```python
from build123d import *

# Parameters (mm, degrees)
SKETCH1_R           = 2.1
BOSS_EXTRUDE1_DEPTH = 5
SKETCH3_W           = 30
SKETCH3_H           = 5
BOSS_EXTRUDE2_DEPTH = 15
FILLET1_R           = 5
SKETCH4_R           = 2.6
CUT_EXTRUDE2_DEPTH  = 108.425323176
FILLET2_R           = 10
SKETCH5_R           = 4.4
CUT_EXTRUDE3_DEPTH  = 108.425323272
SKETCH2_R           = 3.6
CUT_EXTRUDE4_DEPTH  = 114.974558916


with BuildPart() as part:
    # Sketch1 → Boss-Extrude1 (new body)
    with BuildSketch(Plane.XY):
        Polygon((73.634936481, -21), (73.634936481, -20), (103.634936481, -20), (103.634936481, -21), (103.634936481, -45), (73.634936481, -45), align=None)
        with Locations((98.634936481, -35.1)):
            Circle(SKETCH1_R, mode=Mode.SUBTRACT)
        with Locations((78.634936481, -35.1)):
            Circle(SKETCH1_R, mode=Mode.SUBTRACT)
        with Locations((98.634936481, -25.1)):
            Circle(SKETCH1_R, mode=Mode.SUBTRACT)
        with Locations((78.634936481, -25.1)):
            Circle(SKETCH1_R, mode=Mode.SUBTRACT)
    extrude(amount=BOSS_EXTRUDE1_DEPTH)

    # Sketch3 → Boss-Extrude2 (add)
    with BuildSketch(Plane.XY.offset(5)):
        with Locations((88.634936481, -42.5)):
            Rectangle(SKETCH3_W, SKETCH3_H)
    extrude(amount=BOSS_EXTRUDE2_DEPTH)

    # Fillet1
    fillet1_edges = [part.edges().sort_by_distance(p)[0] for p in [
        (103.634936481, -20, 2.5),
        (73.634936481, -20, 2.5),
    ]]
    fillet(fillet1_edges, radius=FILLET1_R)

    # Sketch4 → Cut-Extrude2 (cut, through all)
    with BuildSketch(Plane(origin=(0, -40, 0), x_dir=(1, 0, 0), z_dir=(0, 1, 0))):
        with Locations(Location((88.634936481, -12.5, 0), (0, 0, 180))):
            Circle(SKETCH4_R)
    extrude(amount=-CUT_EXTRUDE2_DEPTH, mode=Mode.SUBTRACT)

    # Fillet2
    # the kernel refuses this fillet: 10 mm, written as the material it adds along each edge
    with BuildSketch(Plane(origin=(73.634936481, -40, 5), x_dir=(0, 1, 0), z_dir=(1, 0, 0))) as fillet2_piece_1_section:
        with BuildLine():
            CenterArc((FILLET2_R, FILLET2_R), FILLET2_R, 180, 90)
            Line((0, FILLET2_R), (0, 0))
            Line((0, 0), (FILLET2_R, 0))
        make_face()
    fillet2_piece_1 = extrude(amount=30, mode=Mode.PRIVATE)
    fillet2_piece_1 = fillet2_piece_1 - Plane(origin=(98.634936481, -35.1, 7.280397509), x_dir=(1, 0, 0), z_dir=(0, 0, -1)) * Cylinder(2.1, 100, mode=Mode.PRIVATE)
    fillet2_piece_1 = fillet2_piece_1 - Plane(origin=(78.634936481, -35.1, 7.280397509), x_dir=(1, 0, 0), z_dir=(0, 0, -1)) * Cylinder(2.1, 100, mode=Mode.PRIVATE)
    fillet2_piece_1 = fillet2_piece_1 - Plane(origin=(88.634936481, -37.846705327, 12.5), x_dir=(-1, 0, 0), z_dir=(0, 1, 0)) * Cylinder(2.6, 100, mode=Mode.PRIVATE)
    add(fillet2_piece_1)

    # Sketch5 → Cut-Extrude3 (cut, through all)
    with BuildSketch(Plane(origin=(0, -40, 0), x_dir=(1, 0, 0), z_dir=(0, 1, 0))):
        with Locations((88.634936481, -12.5)):
            Circle(SKETCH5_R)
    extrude(amount=CUT_EXTRUDE3_DEPTH, mode=Mode.SUBTRACT)

    # Sketch2 → Cut-Extrude4 (cut, through all)
    with BuildSketch(Plane.XY.offset(5)):
        with Locations((98.634936481, -25.1)):
            Circle(SKETCH2_R)
        with Locations(Location((98.634936481, -35.1, 0), (0, 0, 180))):
            Circle(SKETCH2_R)
        with Locations((78.634936481, -25.1)):
            Circle(SKETCH2_R)
        with Locations(Location((78.634936481, -35.1, 0), (0, 0, 180))):
            Circle(SKETCH2_R)
    extrude(amount=CUT_EXTRUDE4_DEPTH, mode=Mode.SUBTRACT)


solid = part.part
```
For this review, take the finished solid that the model builds, in its own axes (mm). A direction names the side the tool comes from. Give positions to 0.01 mm unless a question says otherwise; leave off trailing zeros. Loops run counter-clockwise (first coordinate to the right, second up) from the corner with the lowest first, then second, coordinate; pieces in that order, holes last. Notation, with made-up numbers: M 60,86.25 L 98,86.25 A14 ccw 98,106.25 Z; hole C 28,-7 d8. An arc over 180 degrees is marked long. One line per item, written item: value. Start each with the question number.
Q1. Add section A-A (z = 12.5). Give the boundary of the cut face in (x, y), and give its area (3 significant figures).
Q2. Machinability: for faces 1 (the face through (99.1, -38.67, 6.94)), 2 (the face through (89, -25, 5)), 3 (the face through (96.537, -25.008, 2.465)), which of the approach directions +Z, -Z, +X, -X, +Y, -Y give a long, thin tool a straight path to every point of the face, cutting with its end or side? Answer none if there is none.
Q3. Add section D-D (y = -41). Give the boundary of the cut face in (x, z), and give its area (3 significant figures).
Q4. Draft analysis for pull direction X (two halves, no side actions). For faces 4 (the face through (79.1, -38.67, 6.94)), 5 (the face through (102.209, -21.504, 2.535)), 6 (the face through (73.635, -37, 6)), state which applies: released by +X, released by -X, zero draft, split by the parting line, or undercut.
Q5. For L1, parallel to X at y = -35.1, z = 1.05; L2, parallel to X at y = -33.5, z = 4; L3, parallel to X at y = -41.35, z = 12.5, list the stretches that pass through material, from the lowest coordinate up.
Q6. Add section B-B (x = 77.5). Give the boundary of the cut face in (y, z).
Q7. Add section C-C (y = -35.1). Give the boundary of the cut face in (x, z).
Q8. Clearance check with flat-ended pins moving along their axes: pin 1 Ø4.5 at (x, y) = (78.63, -35.1) entering from +Z; pin 2 Ø1.5 at (x, z) = (94.5, 11.5) entering from +Y; pin 3 Ø4 at (x, z) = (89, 9.5) entering from +Y. State where each tip first meets the part, or that it passes through.
Reply:
1. outline: M 73.63,-45 L 86.03,-45 L 86.03,-40 L 84.23,-40 L 84.23,-39.68 L 73.63,-39.68 Z; M 91.23,-45 L 103.63,-45 L 103.63,-39.68 L 93.03,-39.68 L 93.03,-40 L 91.23,-40 Z
1. area: 131 mm²
2. face 1: +Z
2. face 2: +Z, +X, -X, +Y
2. face 3: +Z, -Z
3. outline: M 73.63,0 L 103.63,0 L 103.63,20 L 73.63,20 Z; hole C 88.63,12.5 d5.2
3. area: 579 mm²
4. face 4: undercut
4. face 5: released by +X
4. face 6: released by -X
5. L1: 73.63 to 76.53, 80.73 to 96.53, 100.73 to 103.63
5. L2: 73.63 to 77.27, 80 to 97.27, 100 to 103.63
5. L3: 73.63 to 86.03, 91.23 to 103.63
6. outline: M -45,0 L -36.87,0 L -36.87,5 L -38.52,5 L -38.52,9.76 A10 cw -40,15 L -40,20 L -45,20 Z; M -33.33,0 L -26.87,0 L -26.87,5 L -30,5 A10 cw -31.68,5.14 L -31.68,5 L -33.33,5 Z; M -23.33,0 L -20.13,0 L -20.13,5 L -23.33,5 Z
7. outline: M 73.63,0 L 76.53,0 L 76.53,5 L 75.03,5 L 75.03,6.4 L 73.63,6.4 Z; M 80.73,0 L 96.53,0 L 96.53,5 L 95.03,5 L 95.03,6.4 L 82.23,6.4 L 82.23,5 L 80.73,5 Z; M 100.73,0 L 103.63,0 L 103.63,6.4 L 102.23,6.4 L 102.23,5 L 100.73,5 Z
8. pin 1: z = 5
8. pin 2: y = -39.05
8. pin 3: y = -36.61
